The model under review builds one solid part; all positions refer to its coordinate system, in mm. A direction names the side the tool comes from. Round coordinates to 2 decimals unless told otherwise and drop trailing zeros. Order: outer loops, then holes, each group sorted by start corner. A loop starts at its lowest first (then second) coordinate and runs counter-clockwise, first axis right, second up. Notation, with made-up numbers: M 23,7 L 77,7 A34 ccw 77,42 Z; hole C 33,-34.5 d7. An arc over 180 degrees is marked long. Answer as a JSON object with one key per item and string values. Group by question number.
1. Clearance check with flat-ended pins moving along their axes: P1, Ø1.5, axis at x = 1.5, y = 2.5, coming from the +Z side; P2, Ø4, axis at x = 0, y = 0, coming from the +Z side; P3, Ø3, axis at y = -2, z = 9.5, coming from the -X side; P4, Ø1.5, axis at x = 0.5, z = 17, coming from the +Y side. State where each tip first meets the part, or that it passes through.
2. Machinability: for faces 5 (the face through (-15, 0, 1.5)), 6 (the face through (-12, 0, 17)), 7 (the face through (-17, 1, 18)), 8 (the face through (-17.5, 0.1, 5.8)), which of the approach directions +Z, -Z, +X, -X, +Y, -Y give a long, thin tool a straight path to every point of the face, cutting with its end or side? Answer none if there is none.
3. To check wall thickness, follow probe 1 along X at (y, z) = (0.25, 6.5); probe 2 along Z at (x, y) = (-6, 2.25); probe 3 along X at (y, z) = (0.5, 10.75). State the ranges of each line that lie inside material, in increasing order. Write a range as [from, to].
4. Add section B-B on z = 4.75. State the section outline as (x, y) points, and give its area (3 significant figures).
5. Mouldability with a two-part tool opening along X and no side actions: class faces 1 (the face through (-19, 0, 12)), 2 (the face through (-7, 4, 12)), 3 (the face through (-2.579, -1.978, 13.324)), 4 (the face through (-10, 0, 10)) as released by +X, released by -X, zero draft, split by the parting line, or undercut.
6. Add section C-C on x = -9.75. State the section outline as (y, z) points, and give its area (3 significant figures).
```python
from build123d import *

# Parameters (mm, degrees)
SKETCH1_R                                           = 4
BOSS_EXTRUDE1_DEPTH                                 = 10
BOSS_EXTRUDE2_DEPTH                                 = 5
SKETCH2_3_R                                         = 2.5
BOSS_EXTRUDE3_DEPTH                                 = 8.5
CBORE_FOR_M3_HEX_SOCKET_HEAD_CAP_SCREW1_D           = 3.6
CBORE_FOR_M3_HEX_SOCKET_HEAD_CAP_SCREW1_CBORE_D     = 6.5
CBORE_FOR_M3_HEX_SOCKET_HEAD_CAP_SCREW1_CBORE_DEPTH = 3.4


with BuildPart() as part:
    # Sketch1 → Boss-Extrude1 (new body)
    with BuildSketch(Plane.XY):
        Circle(SKETCH1_R)
    extrude(amount=BOSS_EXTRUDE1_DEPTH)

    # Sketch2 → Boss-Extrude2 (add)
    with BuildSketch(Plane.XY.offset(10)):
        with BuildLine():
            Line((0, 4), (-15, 4))
            ThreePointArc((-15, 4), (-19, 0), (-15, -4))
            Line((-15, -4), (0, -4))
            ThreePointArc((0, -4), (4, 0), (0, 4))
        make_face()
    extrude(amount=BOSS_EXTRUDE2_DEPTH)

    # Sketch2<3> → Boss-Extrude3 (add)
    with BuildSketch(Plane.XY.offset(10)):
        with Locations((-15, 0)):
            Circle(SKETCH2_3_R)
    extrude(amount=-BOSS_EXTRUDE3_DEPTH)

    # CBORE for M3 Hex Socket Head Cap Screw1 (through all)
    with Locations(Plane.XY.offset(15)):
        with Locations((0, 0)):
            CounterBoreHole(CBORE_FOR_M3_HEX_SOCKET_HEAD_CAP_SCREW1_D / 2, CBORE_FOR_M3_HEX_SOCKET_HEAD_CAP_SCREW1_CBORE_D / 2, CBORE_FOR_M3_HEX_SOCKET_HEAD_CAP_SCREW1_CBORE_DEPTH)

    # Sketch6 → Revolve1 (revolve)
    with BuildSketch(Plane(origin=(0, 0, 0), x_dir=(1, 0, 0), z_dir=(0, 1, 0))):
        Polygon((-15, -15), (-18, -15), (-18, -18), (-16.934791303, -18), (-16.934791303, -20), (-18, -20), (-18, -22), (-15, -22), align=None)
    revolve(axis=Axis((-15, 0, 10), (0, 0, 1)))


solid = part.part
```
Recorded:
{
 "1": {"P1": "stops at z = 15", "P2": "stops at z = 11.6", "P3": "stops at x = -18.96", "P4": "passes through"},
 "2": {"face 5": "-Z, -X, +Y, -Y", "face 6": "+Z", "face 7": "none", "face 8": "-Z"},
 "3": {"probe 1": "x = [-17.49, -12.51], [-3.99, -1.78], [1.78, 3.99]", "probe 2": "z = [10, 15]", "probe 3": "x = [-18.97, -1.73], [1.73, 3.97]"},
 "4": {"outline": "C -15,0 d5; C 0,0 d8; hole C 0,0 d3.6", "area": "59.7 mm²"},
 "5": {"face 1": "released by -X", "face 2": "zero draft", "face 3": "undercut", "face 4": "undercut"},
 "6": {"outline": "M -4,10 L 4,10 L 4,15 L -4,15 Z", "area": "40.0 mm²"}
}
